Geometry: final body of the model. Coordinates: model frame, mm. A direction names the side the tool comes from. Coordinates: 2 decimals unless noted, no trailing zeros. Write each loop counter-clockwise with the first axis right and the second up, starting at its lowest first coordinate (ties: lowest second). Pieces come first, ordered by that corner, then holes. Notation, with made-up numbers: (5, 78) -> (19, 78) arc R21 ccw to (19, 99) -> close; hole circle Ø6 at (-17, 84). An arc over 180 degrees is marked (long way). Answer as a JSON object with one key per item and string values. Group by question number.
```python
from build123d import *

# Parameters (mm, degrees)
F1_DEPTH = 152.4
F2_W     = 19.05
F2_H     = 152.4
F3_DEPTH = 19.05


with BuildPart() as f1:
    # F0 (on Front) → F1 (new body, symmetric)
    with BuildSketch(Plane.XZ):
        Polygon((-375.8118146057, 915.9322428123), (-375.8118146057, 888.9914744491), (513.1796598434, 0), (513.1796598434, 26.9407683632), align=None)
    extrude(amount=F1_DEPTH, both=True)

    # F2 (on face) → F3 (cut)
    with BuildSketch(Plane(origin=(270.0602141033, 0, 270.0602141033), x_dir=(0.7071067812, 0, -0.7071067812), z_dir=(0.7071067812, 0, 0.7071067812))):
        with Locations((264.4478174423, -76.2)):
            Rectangle(F2_W, F2_H)
        with Locations((156.4978174423, -76.2)):
            Rectangle(F2_W, F2_H)
        with Locations((48.5478174423, -76.2)):
            Rectangle(F2_W, F2_H)
        with Locations((-59.4021825577, -76.2)):
            Rectangle(F2_W, F2_H)
        with Locations((-167.3521825577, -76.2)):
            Rectangle(F2_W, F2_H)
        with Locations((-275.3021825577, -76.2)):
            Rectangle(F2_W, F2_H)
        with Locations((-383.2521825577, -76.2)):
            Rectangle(F2_W, F2_H)
        with Locations((-491.2021825577, -76.2)):
            Rectangle(F2_W, F2_H)
        with Locations((-599.1521825577, -76.2)):
            Rectangle(F2_W, F2_H)
        with Locations((-707.1021825577, -76.2)):
            Rectangle(F2_W, F2_H)
        with Locations((-815.0521825577, -76.2)):
            Rectangle(F2_W, F2_H)
    extrude(amount=-F3_DEPTH, mode=Mode.SUBTRACT)


solid = f1.part
```
Item 1: Set-up query: faces 1 (the flat face through (374, 0, 153)), 2 (the flat face through (-120, -152.4, 649)). Return all of +Z, -Z, +X, -X, +Y, -Y with unobstructed straight access to the full face (end or side cutting, diameter ignored); none if empty.
Item 2: Section A-A on y = -34.5. Give the number of separate pieces and of enclosed holes in the cut face, then the cut area to 3 significant figures.
Item 3: Ray query, L1, parallel to X at y = -16, z = 670; L2, parallel to Z at x = 346, y = 124.5; L3, parallel to X at y = -18, z = 50.5. Return the intervals inside material, ascending. Write a range as [from, to].
Item 4: Section B-B on z = 585. Output: boundary loops of the cut face in (x, y), then the cut area to 3 significant figures.
Item 5: Contact query for flat-ended pins moving along their axis: pin 1 (6 mm diameter, centred on y = 73, z = 666.5, fed in from -X); pin 2 (8 mm diameter, centred on x = 453.5, z = 77.5, fed in from -Y); pin 3 (8 mm diameter, centred on x = -318.5, z = 843, fed in from -Y); pin 4 (3 mm diameter, centred on x = 42.5, y = -21.5, fed in from +Z). Output: stop coordinate, or through.
Item 6: Section C-C on y = 42. Output: boundary loops of the cut face in (x, z).
Answer sheet:
{
 "1": {"face 1": "-Y", "face 2": "+Z, -Z, +X, -X, -Y"},
 "2": {"separate pieces": "12", "enclosed holes": "0", "area": "20,000 mm^2"},
 "3": {"L1": "x = [-156.82, -129.88]", "L2": "z = [167.18, 194.12]", "L3": "x = [462.68, 489.62]"},
 "4": {"outline": "(-71.82, -152.4) -> (-44.88, -152.4) -> (-44.88, 152.4) -> (-71.82, 152.4) -> close", "area": "8,210 mm^2"},
 "5": {"pin 1": "stops at x = -156.32", "pin 2": "stops at y = 0", "pin 3": "stops at y = -152.4", "pin 4": "stops at z = 499.12"},
 "6": {"outline": "(-375.81, 888.99) -> (513.18, 0) -> (513.18, 26.94) -> (-375.81, 915.93) -> close"}
}
